Here's how the part is built. I have some questions about the finished solid (model axes, mm). A direction names the side the tool comes from. Give positions to 0.01 mm unless a question says otherwise; leave off trailing zeros. Write each loop counter-clockwise with the first axis right and the second up, starting at its lowest first coordinate (ties: lowest second). Pieces come first, ordered by that corner, then holes. Notation, with made-up numbers: M 50,82 L 64,82 A16 ccw 64,109 Z; hole C 53.5,19 d1. An arc over 180 degrees is marked long. Use one line per item in the form item = value. Start each with the question number.
Autodesk Inventor part; units mm, degrees
ref_plane "YZ Plane" through (0, 0, 0) normal (1, 0, 0) x (0, 1, 0)
ref_plane "XZ Plane" through (0, 0, 0) normal (0, 1, 0) x (-1, 0, 0)
ref_plane "XY Plane" through (0, 0, 0) normal (0, 0, 1) x (1, 0, 0)
sketch "Sketch1" plane through (0, 0, 0) normal (0, 0, 1) x (1, 0, 0)
  circle A0 centre (0, 0) radius 4
  circle A1 centre (0, 0) radius 3.175
  dimension "d0" = 8
  dimension "d1" = 6.35
extrude "Extrusion1" add sketch "Sketch1" along normal blind 1 contours A0 | A1
sketch "Sketch2" plane through (0, 0, 1) normal (0, 0, 1) x (1, 0, 0)
  circle A0 centre (0, 0) radius 4
  circle A1 centre (0, 0) radius 4
  circle A2 centre (0, 0) radius 3.175
  dimension "d4" = 8
  dimension "d5" = 6.35
extrude "Extrusion2" add sketch "Sketch2" along normal blind 2
sketch "Sketch3" plane through (0, 0, 0) normal (0, 0, -1) x (-1, 0, 0)
  circle A0 centre (0, 0) radius 4
  circle A1 centre (0, 0) radius 4
  circle A2 centre (0, 0) radius 3.175
  dimension "d8" = 8
  dimension "d9" = 6.35
extrude "Extrusion3" add sketch "Sketch3" along normal blind 2
properties part number "Pusher.Midplate"
1) Suppose I cut it at C-C, the plane z = 2.5. List the corners of the cut face in (x, y) for me (3 decimals).
2) Please list where these lines run through material, in increasing order: line 1 (Y direction, x = 0, z = 2.25) (3 decimals); line 2 (Z direction, x = -1, y = 2.25); line 3 (X direction, y = -1.5, z = -0.6).
3) Suppose I cut it at A-A, the plane x = 0. List the corners of the cut face in (y, z) for me (3 decimals), and give its area (3 significant figures).
4) On a 3-axis mill with a long thin cutter (end or side, diameter ignored), from which of +Z, -Z, +X, -X, +Y, -Y can I reach the whole of each face in a straight line? I mean faces 3 (the face through (0.69, 3.1, -0.99)), 4 (the face through (0, 0, 1)), 5 (the face through (-3, 2, 3)). Say none if no direction works.
5) Suppose I cut it at D-D, the plane z = 0.8. List the corners of the cut face in (x, y) for me, and give its area (3 significant figures).
6) Will these pins go through, and if not, where does the flat tip stop? P1, Ø1.5, axis at x = 2, y = 0, coming from the +Z side; P2, Ø2, axis at x = 3, z = -0.5, coming from the +Y side; P3, Ø1.5, axis at y = -2, z = 2, coming from the +X side.
7) Thinking about a two-plate mould opening in X: for faces 1 (the face through (3, 2, -2)), 2 (the face through (-0.69, 3.1, 1.99)), which applies, released by +X, released by -X, zero draft, split by the parting line, or undercut?
Checks:
q1.outline = C 0,0 d8; hole C 0,0 d6.35
q2.line_1 = -4 to -3.175, 3.175 to 4
q2.line_2 = 0 to 1
q2.line_3 = -3.71 to -2.8, 2.8 to 3.71
q3.outline = M -4,-2 L -3.175,-2 L -3.175,0 L 3.175,0 L 3.175,-2 L 4,-2 L 4,3 L 3.175,3 L 3.175,1 L -3.175,1 L -3.175,3 L -4,3 Z
q3.area = 14.6 mm^2
q4.face_3 = -Z
q4.face_4 = +Z
q4.face_5 = +Z, +X, -X, +Y, -Y
q5.outline = C 0,0 d8
q5.area = 50.3 mm^2
q6.P1 = 1
q6.P2 = 3.46
q6.P3 = 3.8
q7.face_1 = zero draft
q7.face_2 = undercut
